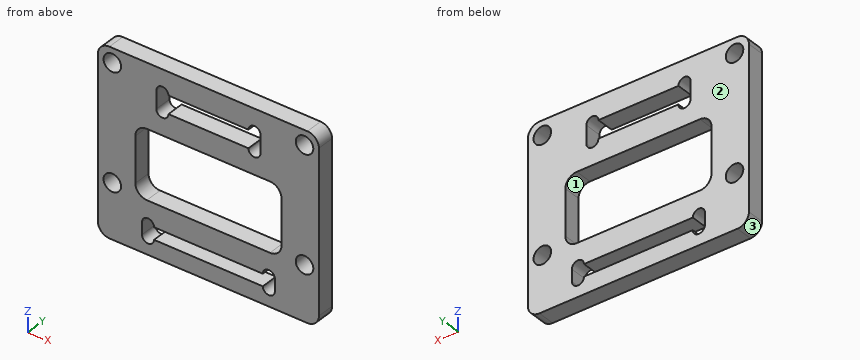
from build123d import *

# Parameters (mm, degrees)
SKETCH_1_W          = 38.4
SKETCH_1_H          = 32
EXTRUDE_1_DEPTH     = 3
SKETCH_2_R          = 1.525
CUT_EXTRUDE_1_DEPTH = 3
SKETCH_3_W          = 23.1
SKETCH_3_H          = 2.1
CUT_EXTRUDE_2_DEPTH = 3
CUT_EXTRUDE_3_DEPTH = 3
SKETCH_5_W          = 18.1
SKETCH_5_H          = 3.1
CUT_EXTRUDE_4_DEPTH = 3
SKETCH_6_R          = 1.05
CUT_EXTRUDE_5_DEPTH = 3
SKETCH_7_W          = 25.4
SKETCH_7_H          = 11.9
CUT_EXTRUDE_6_DEPTH = 3
FILLET_1_R          = 2
FILLET_2_R          = 2


with BuildPart() as part:
    # 草图1 → 凸台-拉伸1 (new body)
    with BuildSketch(Plane(origin=(0, 0, 0), x_dir=(1, 0, 0), z_dir=(0, 1, 0))):
        Rectangle(SKETCH_1_W, SKETCH_1_H)
    extrude(amount=EXTRUDE_1_DEPTH)

    # 草图2 → 切除-拉伸1 (cut)
    with BuildSketch(Plane.XZ):
        with Locations(Location((-16.7, 13.5, 0), (0, 0, 270))):
            Circle(SKETCH_2_R)
        with Locations(Location((16.7, 13.5, 0), (0, 0, 270))):
            Circle(SKETCH_2_R)
        with Locations(Location((-16.7, -6.5, 0), (0, 0, 270))):
            Circle(SKETCH_2_R)
        with Locations(Location((16.7, -6.5, 0), (0, 0, 270))):
            Circle(SKETCH_2_R)
    extrude(amount=-CUT_EXTRUDE_1_DEPTH, mode=Mode.SUBTRACT)

    # 草图3 → 切除-拉伸2 (cut)
    with BuildSketch(Plane.XZ):
        with Locations((0, -12)):
            Rectangle(SKETCH_3_W, SKETCH_3_H)
    extrude(amount=-CUT_EXTRUDE_2_DEPTH, mode=Mode.SUBTRACT)

    # 草图4 → 切除-拉伸3 (cut)
    with BuildSketch(Plane.XZ):
        with BuildLine():
            ThreePointArc((-9.45, -13.05), (-9.75753788, -12.30753788), (-10.5, -12))
            ThreePointArc((-10.5, -12), (-11.24246212, -12.30753788), (-11.55, -13.05))
            Line((-11.55, -13.05), (-9.45, -13.05))
        make_face()
        with BuildLine():
            ThreePointArc((-11.55, -13.05), (-10.5, -14.1), (-9.45, -13.05))
            Line((-9.45, -13.05), (-11.55, -13.05))
        make_face()
        with BuildLine():
            Line((-11.55, -10.95), (-9.45, -10.95))
            ThreePointArc((-9.45, -10.95), (-10.5, -9.9), (-11.55, -10.95))
        make_face()
        with BuildLine():
            ThreePointArc((-10.5, -12), (-9.75753788, -11.69246212), (-9.45, -10.95))
            Line((-9.45, -10.95), (-11.55, -10.95))
            ThreePointArc((-11.55, -10.95), (-11.24246212, -11.69246212), (-10.5, -12))
        make_face()
        with BuildLine():
            Line((9.45, -10.95), (11.55, -10.95))
            ThreePointArc((11.55, -10.95), (10.5, -9.9), (9.45, -10.95))
        make_face()
        with BuildLine():
            ThreePointArc((10.5, -12), (11.24246212, -11.69246212), (11.55, -10.95))
            Line((11.55, -10.95), (9.45, -10.95))
            ThreePointArc((9.45, -10.95), (9.75753788, -11.69246212), (10.5, -12))
        make_face()
        with BuildLine():
            ThreePointArc((11.55, -13.05), (11.24246212, -12.30753788), (10.5, -12))
            ThreePointArc((10.5, -12), (9.75753788, -12.30753788), (9.45, -13.05))
            Line((9.45, -13.05), (11.55, -13.05))
        make_face()
        with BuildLine():
            ThreePointArc((9.45, -13.05), (10.5, -14.1), (11.55, -13.05))
            Line((11.55, -13.05), (9.45, -13.05))
        make_face()
    extrude(amount=-CUT_EXTRUDE_3_DEPTH, mode=Mode.SUBTRACT)

    # 草图5 → 切除-拉伸4 (cut)
    with BuildSketch(Plane.XZ):
        with Locations((0, 10.5)):
            Rectangle(SKETCH_5_W, SKETCH_5_H)
    extrude(amount=-CUT_EXTRUDE_4_DEPTH, mode=Mode.SUBTRACT)

    # 草图6 → 切除-拉伸5 (cut)
    with BuildSketch(Plane.XZ):
        with Locations((-8, 8.95)):
            Circle(SKETCH_6_R)
        with Locations((-8, 12.05)):
            Circle(SKETCH_6_R)
        with Locations((8, 12.05)):
            Circle(SKETCH_6_R)
        with Locations((8, 8.95)):
            Circle(SKETCH_6_R)
    extrude(amount=-CUT_EXTRUDE_5_DEPTH, mode=Mode.SUBTRACT)

    # 草图7 → 切除-拉伸6 (cut)
    with BuildSketch(Plane(origin=(0, 3, 0), x_dir=(1, 0, 0), z_dir=(0, 1, 0))):
        with Locations((0, 1)):
            Rectangle(SKETCH_7_W, SKETCH_7_H)
    extrude(amount=-CUT_EXTRUDE_6_DEPTH, mode=Mode.SUBTRACT)

    # 圆角1
    fillet_1_edges = [part.edges().sort_by_distance(p)[0] for p in [
        (-12.7, 1.5, -6.95),
        (-12.7, 1.5, 4.95),
        (12.7, 1.5, 4.95),
        (12.7, 1.5, -6.95),
    ]]
    fillet(fillet_1_edges, radius=FILLET_1_R)

    # 圆角2
    fillet_2_edges = [part.edges().sort_by_distance(p)[0] for p in [
        (19.2, 1.5, 16),
        (-19.2, 1.5, 16),
        (-19.2, 1.5, -16),
        (19.2, 1.5, -16),
    ]]
    fillet(fillet_2_edges, radius=FILLET_2_R)


solid = part.part
Input: part model. Units: mm. Frame: model coordinates. Face numbers are marked on the shaded views. Coordinates: 2 decimals unless noted, no trailing zeros. Loops run counter-clockwise (first coordinate to the right, second up) from the corner with the lowest first, then second, coordinate; pieces in that order, holes last.
(1) Material intervals for probe 1 along Z at (x, y) = (-4, 1.65); probe 2 along Z at (x, y) = (10.5, 2.6), sorted ascending.
(2) Section C-C on x = -16.7. Return the cut outline in (y, z) (3 decimals).
(3) Section B-B on x = -8. Return the cut outline in (y, z), then the cut area to 3 significant figures.
(4) Pull-direction query (Z, two-part tool) for the marked faces 1, 2 and 3; classes: released by +Z, released by -Z, zero draft, split by the parting line, or undercut.
(5) Section D-D on z = 14.5. Return the cut outline in (x, y).
(6) Section A-A on z = 0. Return the cut outline in (x, y).
Data:
1. probe 1: z = -16 to -13.05, -10.95 to -6.95, 4.95 to 8.95, 12.05 to 16
1. probe 2: z = -16 to -14.1, -9.9 to -6.95, 4.95 to 16
2. outline: (0, -16) - (3, -16) - (3, -8.025) - (0, -8.025) - close; (0, -4.975) - (3, -4.975) - (3, 11.975) - (0, 11.975) - close; (0, 15.025) - (3, 15.025) - (3, 16) - (0, 16) - close
3. outline: (0, -16) - (3, -16) - (3, -13.05) - (0, -13.05) - close; (0, -10.95) - (3, -10.95) - (3, -6.95) - (0, -6.95) - close; (0, 4.95) - (3, 4.95) - (3, 7.9) - (0, 7.9) - close; (0, 13.1) - (3, 13.1) - (3, 16) - (0, 16) - close
3. area: 38.4 mm2
4. face 1: undercut
4. face 2: zero draft
4. face 3: released by -Z
5. outline: (-19.14, 0) - (-17.85, 0) - (-17.85, 3) - (-19.14, 3) - close; (-15.55, 0) - (15.55, 0) - (15.55, 3) - (-15.55, 3) - close; (17.85, 0) - (19.14, 0) - (19.14, 3) - (17.85, 3) - close
6. outline: (-19.2, 0) - (-12.7, 0) - (-12.7, 3) - (-19.2, 3) - close; (12.7, 0) - (19.2, 0) - (19.2, 3) - (12.7, 3) - close
